Can you work these out from the drawing? Everything is in mm from the part's minimum corner. Give positions to 0.01 mm unless a question says otherwise; leave off trailing zeros. Loops run counter-clockwise (first coordinate to the right, second up) from the corner with the lowest first, then second, coordinate; pieces in that order, holes last. Notation, with made-up numbers: (48.25, -19) - (91.25, -19) arc R21 cw to (91.25, -1) - close; hole circle Ø9 at (-1, 54.5). An arc over 180 degrees is marked (long way). One line per item, written item: value. Start each with the question number.
Q1. If I drill on line 1 (X direction, y = 5.75, z = 22.5); line 2 (X direction, y = 4.75, z = 12.5) (3 decimals); line 3 (Z direction, x = 40.5, y = 3.75), over which ranges is the centre line in solid material (lowest first)? Write a range as from..to.
Q2. I want a section at C-C (z = 12.5). Please give me the cut outline in (x, y) (3 decimals).
Q3. I want a section at D-D (y = 9.25). Please give me the cut outline in (x, z) (3 decimals).
Q4. I'm going to push a flat-ended pin straight in: P1, Ø2.5, axis at x = 6.5, z = 22.5, coming from the -Y side. Where does the tip first touch, or does it pass through?
Q5. I want a section at B-B (x = 6.5). Please give me the cut outline in (y, z).
Q6. I want a section at A-A (z = 22.5). Please give me the cut outline in (x, y).
Q7. If we mould it in two halves opening along Z, with no side actions, what happens to the marked faces 1, 2, 3 and 4? For each: released by +Z, released by -Z, zero draft, split by the parting line, or undercut.
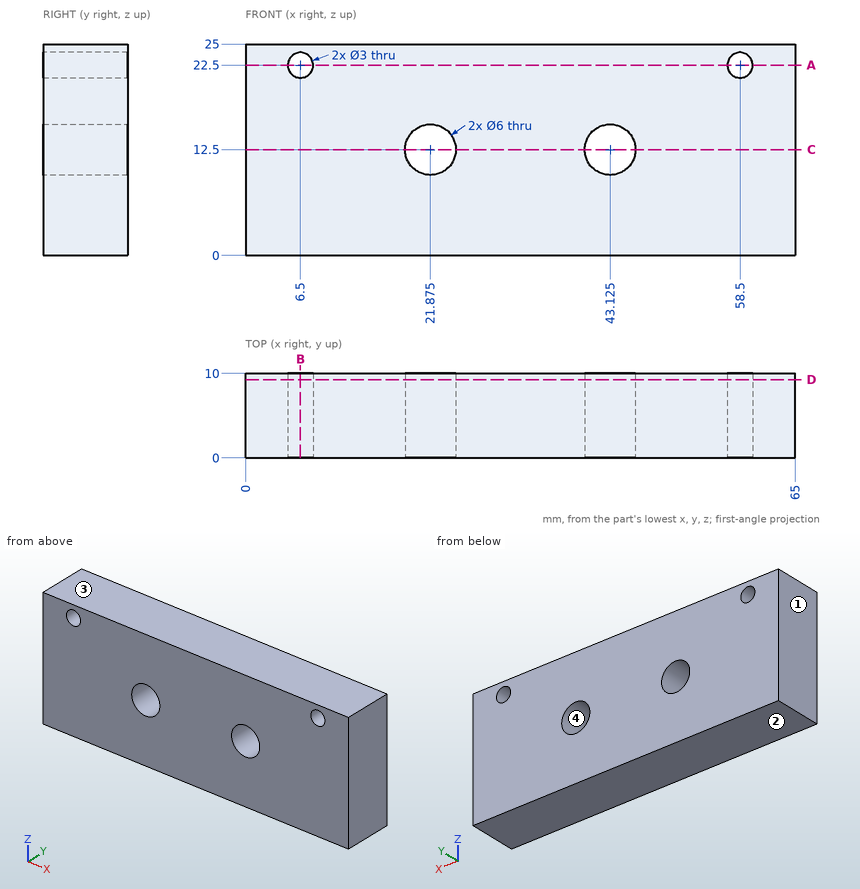
Worked answers:
1. line 1: x = 0..5, 8..57, 60..65
1. line 2: x = 0..18.875, 24.875..40.125, 46.125..65
1. line 3: z = 0..11.05, 13.95..25
2. outline: (0, 0) - (18.875, 0) - (18.875, 10) - (0, 10) - close; (24.875, 0) - (40.125, 0) - (40.125, 10) - (24.875, 10) - close; (46.125, 0) - (65, 0) - (65, 10) - (46.125, 10) - close
3. outline: (0, 0) - (65, 0) - (65, 25) - (0, 25) - close; hole circle Ø3 at (6.5, 22.5); hole circle Ø6 at (21.875, 12.5); hole circle Ø6 at (43.125, 12.5); hole circle Ø3 at (58.5, 22.5)
4. P1: passes through
5. outline: (0, 0) - (10, 0) - (10, 21) - (0, 21) - close; (0, 24) - (10, 24) - (10, 25) - (0, 25) - close
6. outline: (0, 0) - (5, 0) - (5, 10) - (0, 10) - close; (8, 0) - (57, 0) - (57, 10) - (8, 10) - close; (60, 0) - (65, 0) - (65, 10) - (60, 10) - close
7. face 1: zero draft
7. face 2: released by -Z
7. face 3: released by +Z
7. face 4: undercut
